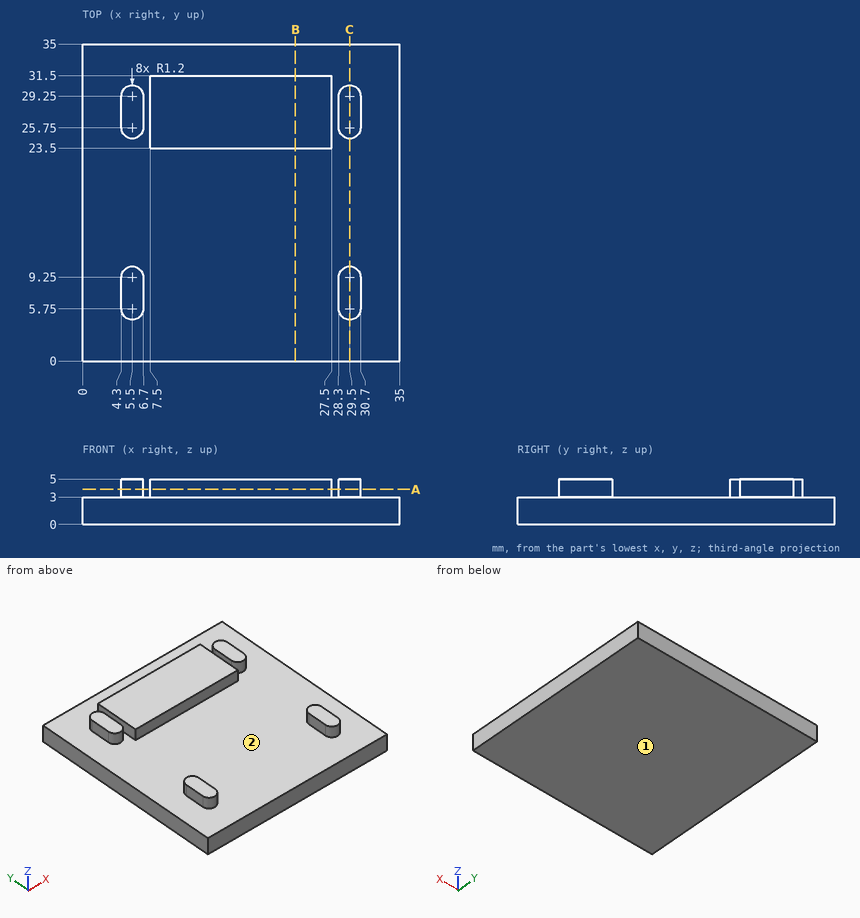
The drawing under review shows one solid part. Ordinate dimensions are in mm from its lowest x, y, z. Coordinates: 2 decimals unless noted, no trailing zeros. Order: outer loops, then holes, each group sorted by start corner. A loop starts at its lowest first (then second) coordinate and runs counter-clockwise, first axis right, second up. Notation, with made-up numbers: (-39, 52) -> (-21, 52) arc R19 ccw to (-21, 75) -> close; hole circle Ø8 at (-16.5, 55.25). An arc over 180 degrees is marked (long way). Answer in a Markdown table with one row per item. Add a question column.
Item 1: We need section A-A on z = 3.85. Write out the cut boundary in (x, y), plus the area to 3 significant figures.
Item 2: To check wall thickness, follow probe 1 along X at (y, z) = (26, 3.6); probe 2 along Y at (x, z) = (19, 3.55); probe 3 along Z at (x, y) = (6, 3). State the ranges of each line that lie inside material, in increasing order.
Item 3: Mouldability with a two-part tool opening along X and no side actions: class the marked faces 1 and 2 as +X half, -X half, draft (parallel to the pull), parting line (faces both ways), or undercut.
Item 4: We need section B-B on x = 23.5. Write out the cut boundary in (y, z), plus the area to 3 significant figures.
Item 5: Clearance check with flat-ended pins moving along their axes: pin 1 (2 mm diameter, centred on y = 27.5, z = 4.5, fed in from +X); pin 2 (0.6 mm diameter, centred on y = 26, z = 4, fed in from -X); pin 3 (1.6 mm diameter, centred on x = 15.5, z = 4, fed in from -Y). State where each tip first meets the part, or that it passes through.
Item 6: We need section C-C on x = 29.5. Write out the cut boundary in (y, z).
Final values:
| question | item | result |
|---|---|---|
| 1 | outline | (4.3, 5.75) arc R1.2 ccw to (6.7, 5.75) -> (6.7, 9.25) arc R1.2 ccw to (4.3, 9.25) -> close; (4.3, 25.75) arc R1.2 ccw to (6.7, 25.75) -> (6.7, 29.25) arc R1.2 ccw to (4.3, 29.25) -> close; (7.5, 23.5) -> (27.5, 23.5) -> (27.5, 31.5) -> (7.5, 31.5) -> close; (28.3, 5.75) arc R1.2 ccw to (30.7, 5.75) -> (30.7, 9.25) arc R1.2 ccw to (28.3, 9.25) -> close; (28.3, 25.75) arc R1.2 ccw to (30.7, 25.75) -> (30.7, 29.25) arc R1.2 ccw to (28.3, 29.25) -> close |
| 1 | area | 212 mm2 |
| 2 | probe 1 | x = 4.3 to 6.7, 7.5 to 27.5, 28.3 to 30.7 |
| 2 | probe 2 | y = 23.5 to 31.5 |
| 2 | probe 3 | z = 0 to 3 |
| 3 | face 1 | draft |
| 3 | face 2 | undercut |
| 4 | outline | (0, 0) -> (35, 0) -> (35, 3) -> (31.5, 3) -> (31.5, 5) -> (23.5, 5) -> (23.5, 3) -> (0, 3) -> close |
| 4 | area | 121 mm2 |
| 5 | pin 1 | stops at x = 30.7 |
| 5 | pin 2 | stops at x = 4.3 |
| 5 | pin 3 | stops at y = 23.5 |
| 6 | outline | (0, 0) -> (35, 0) -> (35, 3) -> (30.45, 3) -> (30.45, 5) -> (24.55, 5) -> (24.55, 3) -> (10.45, 3) -> (10.45, 5) -> (4.55, 5) -> (4.55, 3) -> (0, 3) -> close |
